Part print with two shaded views. Sizes in mm from the minimum x, y, z corner. Coordinates: 2 decimals unless noted, no trailing zeros. Order: outer loops, then holes, each group sorted by start corner. A loop starts at its lowest first (then second) coordinate and runs counter-clockwise, first axis right, second up. Notation, with made-up numbers: (81.25, 17) - (88.25, 17) arc R15 ccw to (88.25, 40) - close; hole circle Ø7 at (7.5, 39.5). An arc over 180 degrees is marked (long way). Return JSON: item names as keys, results as strings.
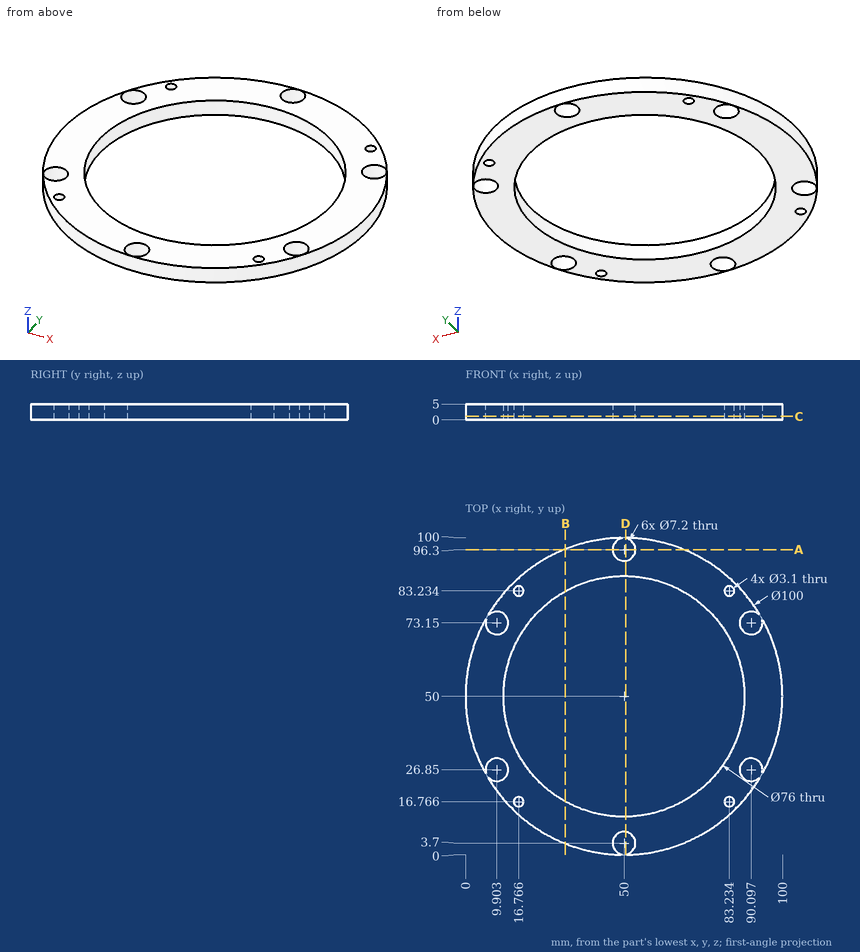
Item 1: Band-saw the part on D-D, the plane x = 50.5. List the corners of the cut face in (y, z).
Findings below:
{"outline": "(0, 0) - (0.13, 0) - (0.13, 5) - (0, 5) - close; (7.27, 0) - (12, 0) - (12, 5) - (7.27, 5) - close; (88, 0) - (92.73, 0) - (92.73, 5) - (88, 5) - close; (99.87, 0) - (100, 0) - (100, 5) - (99.87, 5) - close"}
Item 2: Drop a flat-ended pin along its axis: P1, Ø2, axis at x = 56.5, z = 1.5, coming from the -Y side. Give the stop position or say it passes through.
Findings below:
{"P1": "stops at y = 0.3"}
Item 3: Wall check: L1, parallel to Y at x = 9, z = 0.9 (3 decimals); L2, parallel to X at y = 17.5, z = 1.45; L3, parallel to X at y = 29, z = 1.65. Give the ranges that are in metal, low to high. Write a range as [from, to].
Findings below:
{"L1": "y = [21.382, 23.365], [30.335, 69.665], [76.635, 78.618]", "L2": "x = [12, 15.4], [18.13, 30.31], [69.69, 81.87], [84.6, 88]", "L3": "x = [4.62, 7.02], [12.79, 18.33], [81.67, 87.21], [92.98, 95.38]"}
Item 4: Band-saw the part on B-B, the plane x = 31.5. List the corners of the cut face in (y, z), then the cut area to 3 significant figures.
Findings below:
{"outline": "(3.55, 0) - (16.81, 0) - (16.81, 5) - (3.55, 5) - close; (83.19, 0) - (96.45, 0) - (96.45, 5) - (83.19, 5) - close", "area": "133 mm²"}
Item 5: Band-saw the part on C-C, the plane z = 1.1. Count the separate pieces of the cut face and the enclosed holes in it, then the cut area to 3 significant figures.
Findings below:
{"separate pieces": "1", "enclosed holes": "11", "area": "3,040 mm²"}
Item 6: Band-saw the part on A-A, the plane y = 96.3. List the corners of the cut face in (x, z).
Findings below:
{"outline": "(31.12, 0) - (46.4, 0) - (46.4, 5) - (31.12, 5) - close; (53.6, 0) - (68.88, 0) - (68.88, 5) - (53.6, 5) - close"}
